```python
from build123d import *

# Parameters (mm, degrees)
SKETCH2_W           = 25.4
SKETCH2_H           = 25.4
BOSS_EXTRUDE1_DEPTH = 304.8
SKETCH4_W           = 19.05
SKETCH4_H           = 19.05
CUT_EXTRUDE1_DEPTH  = 306.328708116
SKETCH5_R           = 3.2639
CUT_EXTRUDE2_DEPTH  = 304.8
SKETCH6_R           = 3.2639
CUT_EXTRUDE3_DEPTH  = 304.8
SKETCH8_R           = 3.2639
CUT_EXTRUDE5_DEPTH  = 307.120058147
SKETCH9_R           = 3.2639
CUT_EXTRUDE6_DEPTH  = 307.120058147
SKETCH10_R          = 3.2639
CUT_EXTRUDE7_DEPTH  = 307.120058147


with BuildPart() as part:
    # Sketch2 → Boss-Extrude1 (new body)
    with BuildSketch(Plane.XY):
        Rectangle(SKETCH2_W, SKETCH2_H)
    extrude(amount=BOSS_EXTRUDE1_DEPTH)

    # Sketch4 → Cut-Extrude1 (cut, through all)
    with BuildSketch(Plane.XY):
        Rectangle(SKETCH4_W, SKETCH4_H)
    extrude(amount=CUT_EXTRUDE1_DEPTH, mode=Mode.SUBTRACT)

    # Sketch5 → Cut-Extrude2 (cut)
    with BuildSketch(Plane(origin=(0, 12.7, 0), x_dir=(1, 0, 0), z_dir=(0, 1, 0))):
        with Locations(Location((2.54, -12.7, 0), (0, 0, 270))):
            Circle(SKETCH5_R)
    extrude(amount=-CUT_EXTRUDE2_DEPTH, mode=Mode.SUBTRACT)

    # Sketch6 → Cut-Extrude3 (cut)
    with BuildSketch(Plane(origin=(0, 12.7, 0), x_dir=(1, 0, 0), z_dir=(0, 1, 0))):
        with Locations(Location((2.54, -62.738, 0), (0, 0, 270))):
            Circle(SKETCH6_R)
    extrude(amount=-CUT_EXTRUDE3_DEPTH, mode=Mode.SUBTRACT)

    # Sketch8 → Cut-Extrude5 (cut, through all)
    with BuildSketch(Plane.ZY.offset(12.7)):
        with Locations((292.1, 0)):
            Circle(SKETCH8_R)
    extrude(amount=-CUT_EXTRUDE5_DEPTH, mode=Mode.SUBTRACT)

    # Sketch9 → Cut-Extrude6 (cut, through all)
    with BuildSketch(Plane(origin=(12.7, 0, 0), x_dir=(0, 0, -1), z_dir=(1, 0, 0))):
        with Locations((-228.6, 0)):
            Circle(SKETCH9_R)
    extrude(amount=-CUT_EXTRUDE6_DEPTH, mode=Mode.SUBTRACT)

    # Sketch10 → Cut-Extrude7 (cut, through all)
    with BuildSketch(Plane.ZY.offset(12.7)):
        with Locations((120.65, 0)):
            Circle(SKETCH10_R)
    extrude(amount=-CUT_EXTRUDE7_DEPTH, mode=Mode.SUBTRACT)


solid = part.part
```
Build history of the part. All positions in model axes, mm. A direction names the side the tool comes from. Give positions to 0.01 mm unless a question says otherwise; leave off trailing zeros. Loops run counter-clockwise (first coordinate to the right, second up) from the corner with the lowest first, then second, coordinate; pieces in that order, holes last.
Item 1: Pull direction Y, two halves, no side cores. Call faces 1 (the face through (0, -12.7, 150)), 2 (the face through (0, 12.7, 150)), 3 (the face through (2.68, -11.09, 9.44)), 4 (the face through (-9.525, 0, 150)): released by +Y, released by -Y, zero draft, split by the parting line, or undercut.
Answers follow:
face 1: released by -Y
face 2: released by +Y
face 3: zero draft
face 4: undercut
Item 2: Flat gauge pin, fed straight in: pin 1 (5 mm diameter, centred on x = 2.54, z = 62.738, fed in from +Y) (3 decimals). Where does the tip first touch, or does it go through?
Answers follow:
pin 1: passes through
Item 3: Which spindle directions (+Z, -Z, +X, -X, +Y, -Y) get a long thin tool onto all of the face, cutting with end or side? Do faces 5 (the face through (0, -9.525, 150)), 6 (the face through (3.52, -11.09, 65.85)). Say none if no direction does.
Answers follow:
face 5: +Z, -Z
face 6: +Y, -Y
Item 4: Drill centre lines: line 1 (X direction, y = 2.5, z = 264.5) (3 decimals); line 2 (Y direction, x = 10.4, z = 228.6). Where is each one in solid material? Low to high.
Answers follow:
line 1: x = -12.7 to -9.525, 9.525 to 12.7
line 2: y = -12.7 to -3.26, 3.26 to 12.7
Item 5: Slice it at A-A, the plane y = -5.75. List the corners of the cut face in (x, z) (3 decimals), and give its area (3 significant figures).
Answers follow:
outline: (-12.7, 0) - (-9.525, 0) - (-9.525, 304.8) - (-12.7, 304.8) - close; (9.525, 0) - (12.7, 0) - (12.7, 304.8) - (9.525, 304.8) - close
area: 1,940 mm2
Item 6: Slice it at B-B, the plane z = 99. List the corners of the cut face in (x, y) (3 decimals), and give its area (3 significant figures).
Answers follow:
outline: (-12.7, -12.7) - (12.7, -12.7) - (12.7, 12.7) - (-12.7, 12.7) - close; hole (-9.525, -9.525) - (9.525, -9.525) - (9.525, 9.525) - (-9.525, 9.525) - close
area: 282 mm2
Item 7: Slice it at C-C, the plane z = 292.1. List the corners of the cut face in (x, y) (3 decimals).
Answers follow:
outline: (-12.7, -12.7) - (12.7, -12.7) - (12.7, -3.264) - (9.525, -3.264) - (9.525, -9.525) - (-9.525, -9.525) - (-9.525, -3.264) - (-12.7, -3.264) - close; (-12.7, 3.264) - (-9.525, 3.264) - (-9.525, 9.525) - (9.525, 9.525) - (9.525, 3.264) - (12.7, 3.264) - (12.7, 12.7) - (-12.7, 12.7) - close
